CAD build for the part. Positions are in the model's coordinates, mm. Face numbers are marked on the shaded views. A direction names the side the tool comes from. Give positions to 0.01 mm unless a question says otherwise; leave off trailing zeros. Write each loop counter-clockwise with the first axis right and the second up, starting at its lowest first coordinate (ties: lowest second). Pieces come first, ordered by that corner, then holes. Notation, with made-up numbers: (74.5, -5.5) - (132.5, -5.5) arc R15 ccw to (132.5, 10.5) - close; hole circle Ø5 at (-40, -22). An arc over 180 degrees is marked (long way). Answer as a JSON object with one key per item and string values.
from build123d import *

# Parameters (mm, degrees)
SKETCH1_R                       = 50
BOSS_EXTRUDE1_DEPTH             = 26
SKETCH2_R                       = 42
CUT_EXTRUDE1_DEPTH              = 5
SKETCH3_R                       = 5
HUB_DISTANCE_TO_WORK_WITH_DEPTH = 10


with BuildPart() as part:
    # Sketch1 → Boss-Extrude1 (new body)
    with BuildSketch(Plane(origin=(0, 0, 0), x_dir=(1, 0, 0), z_dir=(0, 1, 0))):
        Circle(SKETCH1_R)
    extrude(amount=BOSS_EXTRUDE1_DEPTH)

    # Sketch2 → Cut-Extrude1 (cut)
    with BuildSketch(Plane(origin=(0, 26, 0), x_dir=(1, 0, 0), z_dir=(0, 1, 0))):
        Circle(SKETCH2_R)
    extrude(amount=-CUT_EXTRUDE1_DEPTH, mode=Mode.SUBTRACT)

    # Sketch3 → hub_distance_to_work_with (add)
    with BuildSketch(Plane.XZ):
        Circle(SKETCH3_R)
    extrude(amount=HUB_DISTANCE_TO_WORK_WITH_DEPTH)


solid = part.part
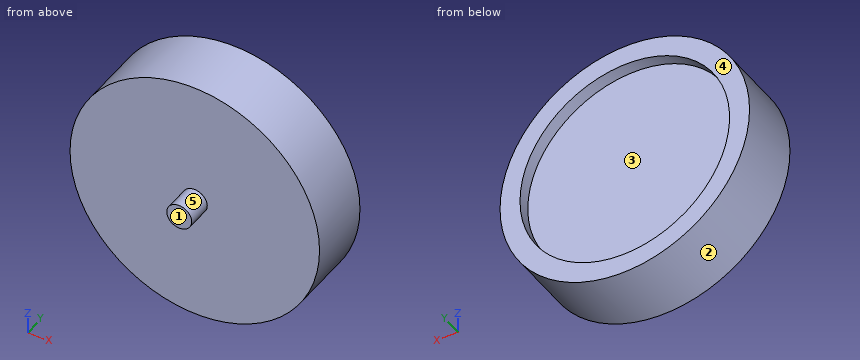
(1) Saw through at C-C, the plane y = -6.5. Give the cut face in (x, z).
Answer key:
{"outline": "circle Ø10 at (0, 0)"}
(2) Flat gauge pins, fed straight in: P1, Ø1, axis at x = 2, y = 4, coming from the -Z side; P2, Ø10, axis at x = -16, z = 13.5, coming from the +Y side; P3, Ø6, axis at x = -19.5, z = 37.5, coming from the -Y side; P4, Ø3, axis at x = -7, y = -2, coming from the -Z side (1 decimal). Where does each tip first touch, or does it go through?
Answer key:
{"P1": "stops at z = -49.98", "P2": "stops at y = 21", "P3": "stops at y = 0", "P4": "passes through"}
(3) Probe L1, parallel to Z at x = 0, y = 22.8; L2, parallel to Y at x = 12, z = 25.5. List the from-to ranges inside material, lowest first. Write a range as [from, to].
Answer key:
{"L1": "z = [-50, -42], [42, 50]", "L2": "y = [0, 21]"}
(4) Pull direction X, two halves, no side cores. Call the marked faces 1, 2 and 3: pulls with the +X half, pulls with the -X half, needs draft (parallel to the pull), parting line crosses it, or undercut.
Answer key:
{"face 1": "needs draft", "face 2": "parting line crosses it", "face 3": "undercut"}
(5) Saw through at B-B, the plane x = 0. Give the cut face in (y, z), and give its area (3 significant figures).
Answer key:
{"outline": "(-10, -5) - (0, -5) - (0, -50) - (26, -50) - (26, -42) - (21, -42) - (21, 42) - (26, 42) - (26, 50) - (0, 50) - (0, 5) - (-10, 5) - close", "area": "2,280 mm²"}
(6) Saw through at A-A, the plane z = 0. Give the cut face in (x, y).
Answer key:
{"outline": "(-50, 0) - (-5, 0) - (-5, -10) - (5, -10) - (5, 0) - (50, 0) - (50, 26) - (42, 26) - (42, 21) - (-42, 21) - (-42, 26) - (-50, 26) - close"}
(7) Saw through at D-D, the plane z = 11. Give the cut face in (x, y) (3 decimals).
Answer key:
{"outline": "(-48.775, 0) - (48.775, 0) - (48.775, 26) - (40.534, 26) - (40.534, 21) - (-40.534, 21) - (-40.534, 26) - (-48.775, 26) - close"}
(8) 3-axis set-ups, long thin cutter, end or side, ignore diameter. For the marked faces 4 and 5: which of +Z, -Z, +X, -X, +Y, -Y reach the whole face in a straight line?
Answer key:
{"face 4": "+Z, -Z, +X, -X, +Y", "face 5": "-Y"}
